Solid Edge part; units mm, degrees
sketch "Sketch1" plane through (0, 0, 0) normal (0, 0, 1) x (1, 0, 0)
  line L0 (233.3222, 117.1952) -> (-118.1099, -234.2368)
  line L1 (-118.1099, -234.2368) -> (-153.4653, -198.8815)
  line L2 (-153.4653, -198.8815) -> (-153.4653, -24.9332)
  line L3 (-153.4653, -24.9332) -> (24.0185, 152.5506)
  line L4 (24.0185, 152.5506) -> (197.9668, 152.5506)
  line L5 (197.9668, 152.5506) -> (233.3222, 117.1952)
  circle A0 centre (-133.4653, -62.7673) radius 2.9988
  circle A1 centre (-133.4653, -162.7673) radius 2.9988
  circle A2 centre (60.674, 131.0545) radius 2.9988
  circle A3 centre (160.674, 131.0545) radius 2.9988
  dimension "D1" = 233.3222
  dimension "D2" = 197.9668
  dimension "D3" = 133.4653
  dimension "D4" = 60.674
  dimension "D5" = 60.674
  dimension "D6" = 197.9668
extrude "Protrusion1" add sketch "Sketch1" along normal blind 3
sketch "Sketch2" plane through (215.6445, 134.8729, 1.5) normal (0.7071068, 0.7071068, 0) x (0.7071068, -0.7071068, 0)
  line L0 (-25, 1.5) -> (25, 1.5)
  line L1 (25, 1.5) -> (25, -1.5)
  line L2 (25, -1.5) -> (-25, -1.5)
  line L3 (-25, -1.5) -> (-25, 1.5)
extrude "Extrusionsausprägung_2" add sketch "Sketch2" along normal blind 5.83
sketch "Sketch3" plane through (-135.7876, -216.5592, 1.5) normal (-0.7071068, -0.7071068, 0) x (0.7071068, -0.7071068, 0)
  line L0 (-25, 1.5) -> (25, 1.5)
  line L1 (25, 1.5) -> (25, -1.5)
  line L2 (25, -1.5) -> (-25, -1.5)
  line L3 (-25, -1.5) -> (-25, 1.5)
extrude "Extrusionsausprägung_3" add sketch "Sketch3" along normal blind 7.9
sketch "Sketch4" plane through (-64.7234, 63.8087, 1.5) normal (-0.7071068, 0.7071068, 0) x (-0.7071068, -0.7071068, 0)
  line L0 (-125.5, 1.5) -> (125.5, 1.5)
  line L1 (125.5, 1.5) -> (125.5, -1.5)
  line L2 (125.5, -1.5) -> (-125.5, -1.5)
  line L3 (-125.5, -1.5) -> (-125.5, 1.5)
extrude "Extrusionsausprägung_4" add sketch "Sketch4" along normal blind 7.07
sketch "Sketch5" plane through (39.1294, -41.2038, 3) normal (0, 0, 1) x (1, 0, 0)
  line L0 (-197.5939, 21.2698) -> (-192.5947, 16.2705)
  line L1 (-192.5947, 16.2705) -> (-192.5947, -157.6777)
  line L2 (-192.5947, -157.6777) -> (-198.1808, -163.2639)
  arc A0 (-198.1808, -163.2639) -> (-197.5939, 21.2698) centre (-106.2037, -71.2887) cw
extrude "Protrusion2" add sketch "Sketch5" against normal up to vertex (3 mm away)
sketch "Sketch6" plane through (20.0805, -41.2038, 3) normal (0, 0, 1) x (1, 0, 0)
  line L0 (-1.0612, 198.7536) -> (3.938, 193.7543)
  line L1 (3.938, 193.7543) -> (177.8863, 193.7543)
  line L2 (177.8863, 193.7543) -> (182.0087, 197.8768)
  arc A0 (-1.0612, 198.7536) -> (182.0087, 197.8768) centre (90.0395, 107.6528) cw
extrude "Protrusion3" add sketch "Sketch6" against normal up to vertex (3 mm away)
properties material "Nylon, allgemein"
Check sheet for the modelled part. Datum: model origin and axes. Units: mm. Round coordinates to 2 decimals unless told otherwise and drop trailing zeros. Write each loop counter-clockwise with the first axis right and the second up, starting at its lowest first coordinate (ties: lowest second). Pieces come first, ordered by that corner, then holes. Notation, with made-up numbers: (10.5, 67) - (69.5, 67) arc R18 cw to (69.5, 76) - close; hole circle Ø6 at (-1.75, 49.25). An arc over 180 degrees is marked (long way). Return JSON: item names as keys, results as strings.
Q1. Cross-section at B-B (y = -49). Record the boundary of the cut face in (x, z), then the cut area to 3 significant figures.
Returned:
{"outline": "(-180.6, 0) - (67.13, 0) - (67.13, 3) - (-180.6, 3) - close", "area": "743 mm²"}
Q2. Cross-section at C-C (x = 87). Record the boundary of the cut face in (y, z), then the cut area to 3 significant figures.
Returned:
{"outline": "(-29.13, 0) - (193.19, 0) - (193.19, 3) - (-29.13, 3) - close", "area": "667 mm²"}
Q3. Cross-section at A-A (z = 0.75). Record the boundary of the cut face in (x, y).
Returned:
{"outline": "(-159.05, -204.47) - (-123.7, -239.82) - (-118.11, -234.24) - (233.32, 117.2) - (237.44, 121.32) - (202.09, 156.67) arc R128.84 ccw to (19.02, 157.55) - (-158.46, -19.93) arc R130.07 ccw to start; hole circle Ø6 at (-133.47, -162.77); hole circle Ø6 at (-133.47, -62.77); hole circle Ø6 at (60.67, 131.05); hole circle Ø6 at (160.67, 131.05)"}
Q4. Scan lines: L1, parallel to Y at x = -131, z = 2.7; L2, parallel to X at y = -162, z = 0.3; L3, parallel to X at y = 85, z = 2.5. Record each from-to range of solid material in increasing order. Write a range as from..to.
Returned:
{"L1": "y = -232.52..-164.47, -161.06..-64.47, -61.06..7.53", "L2": "x = -187.36..-136.36, -130.57..-45.87", "L3": "x = -53.53..201.13"}
Q5. Depth check by flat-ended pin: P1, Ø1, axis at y = 8, z = 2.5, coming from the -X side; P2, Ø1.5, axis at y = -170, z = 1.5, coming from the +X side. Enter the tip coordinate at first touch or a pass-through.
Returned:
{"P1": "stops at x = -131.03", "P2": "stops at x = -53.12"}
